Can you work these out from the model? Positions are in its coordinate system, mm. A direction names the side the tool comes from. Coordinates: 2 decimals unless noted, no trailing zeros. Order: outer loops, then holes, each group sorted by start corner. A loop starts at its lowest first (then second) coordinate and runs counter-clockwise, first axis right, second up. Notation, with made-up numbers: (72, 5.25) -> (81, 5.25) arc R30 ccw to (81, 31.25) -> close; hole circle Ø7 at (41.5, 2). An arc over 180 degrees is marked (long way). Use a Markdown table: item, result. Add a question column.
1. If I drill on line 1 along X through (y, z) = (46.5, -4); line 2 along Z through (x, y) = (-49, 14.5); line 3 along Z through (x, y) = (-22, 29), over which ranges is the centre line in solid material (lowest first)? Write a range as from..to.
2. We'd pull the mould along Y, two halves only. Please class faces 6 (the flat face through (-11, 0, -11)), 7 (the flat face through (49.429, 25, -9)), 8 (the flat face through (-22.3, 28.2, -58.583)): pulls with the +Y half, pulls with the -Y half, needs draft (parallel to the pull), parting line crosses it, or undercut.
3. For faces 1 (the flat face through (-70.571, 25, -9)), 2 (the cylindrical face through (-13.173, 12.785, -59.322)), 3 (the flat face through (-11, 25, 39.917)), 4 (the flat face through (-66.571, 27, -9)), 5 (the flat face through (-11, 40, -57)), which set-ups out of +Z, -Z, +X, -X, +Y, -Y let a thin tool reach every point of the face, with its end or its side?
4. Suppose I cut it at A-A, the plane x = 11.5. List the corners of the cut face in (y, z) for me.
5. For pin 1 Ø1.5 at (x, y) = (30.5, 26.5) entering from -Z; pin 2 Ø2 at (x, z) = (-55.5, -14) entering from +Y; pin 3 Ø1.5 at (x, z) = (-49, 17.5) entering from +Y, each with a flat end and sliding along its axis, tell me the tip position at first contact or that it passes through.
6. Suppose I cut it at B-B, the plane y = 23. List the corners of the cut face in (x, z) for me, then the cut area to 3 significant figures.
7. Suppose I cut it at D-D, the plane x = -14. List the corners of the cut face in (y, z) for me, then the cut area to 3 significant figures.
8. Suppose I cut it at C-C, the plane z = -38. List the corners of the cut face in (x, y) for me.
```python
from build123d import *

# Parameters (mm, degrees)
SKETCH1_W           = 120
SKETCH1_H           = 100
BOSS_EXTRUDE1_DEPTH = 50
SKETCH2_W           = 112
SKETCH2_H           = 92
CUT_EXTRUDE1_DEPTH  = 46
SKETCH3_W           = 28
SKETCH3_H           = 70
BOSS_EXTRUDE3_DEPTH = 8
SKETCH6_W           = 24.21
SKETCH6_H           = 8
CUT_EXTRUDE4_DEPTH  = 66
CUT_EXTRUDE6_DEPTH  = 66
SKETCH8_W           = 26
SKETCH8_H           = 31
CUT_EXTRUDE7_DEPTH  = 2.5
SKETCH9_R           = 12
CUT_EXTRUDE8_DEPTH  = 2.5
SKETCH10_R          = 7
CUT_EXTRUDE9_DEPTH  = 12.5


with BuildPart() as part:
    # Sketch1 → Boss-Extrude1 (new body)
    with BuildSketch(Plane(origin=(0, 0, 0), x_dir=(1, 0, 0), z_dir=(0, 1, 0))):
        with Locations((-10.571222942, 10.082692781)):
            Rectangle(SKETCH1_W, SKETCH1_H)
    extrude(amount=BOSS_EXTRUDE1_DEPTH)

    # Sketch2 → Cut-Extrude1 (cut)
    with BuildSketch(Plane(origin=(0, 50, 0), x_dir=(1, 0, 0), z_dir=(0, 1, 0))):
        with Locations((-10.571222942, 10.082692781)):
            Rectangle(SKETCH2_W, SKETCH2_H)
    extrude(amount=-CUT_EXTRUDE1_DEPTH, mode=Mode.SUBTRACT)

    # Sketch3 → Boss-Extrude3 (add)
    with BuildSketch(Plane(origin=(0, 4, 0), x_dir=(1, 0, 0), z_dir=(0, 1, 0))):
        with Locations((-42.571222942, 25.082692781)):
            Rectangle(SKETCH3_W, SKETCH3_H)
    extrude(amount=BOSS_EXTRUDE3_DEPTH)

    # Sketch6 → Cut-Extrude4 (cut)
    with BuildSketch(Plane.XY.offset(9.917307219)):
        with Locations((-42.569304131, 8)):
            Rectangle(SKETCH6_W, SKETCH6_H)
    extrude(amount=-CUT_EXTRUDE4_DEPTH, mode=Mode.SUBTRACT)

    # Sketch7 → Cut-Extrude6 (cut)
    with BuildSketch(Plane.XY.offset(-56.082692781)):
        Polygon((-54.674304131, 12), (-50.474304131, 12), (-50.474304131, 6.53), (-47.074304131, 6.53), (-47.074304131, 12), (-38.074304131, 12), (-38.074304131, 6.53), (-34.664304131, 6.53), (-34.664304131, 12), (-30.464304131, 12), (-30.464304131, 6.53), (-30.464304131, 4), (-54.674304131, 4), (-54.674304131, 6.53), align=None)
    extrude(amount=-CUT_EXTRUDE6_DEPTH, mode=Mode.SUBTRACT)

    # Sketch8 → Cut-Extrude7 (cut)
    with BuildSketch(Plane.XY.offset(-56.082692781)):
        with Locations((-10.571222942, 24.5)):
            Rectangle(SKETCH8_W, SKETCH8_H)
    extrude(amount=-CUT_EXTRUDE7_DEPTH, mode=Mode.SUBTRACT)

    # Sketch9 → Cut-Extrude8 (cut)
    with BuildSketch(Plane.XY.offset(-58.582692781)):
        with Locations((-10.571222942, 24.5)):
            Circle(SKETCH9_R)
    extrude(amount=-CUT_EXTRUDE8_DEPTH, mode=Mode.SUBTRACT)

    # Sketch10 → Cut-Extrude9 (cut)
    with BuildSketch(Plane(origin=(0, 0, -60.082692781), x_dir=(-1, 0, 0), z_dir=(0, 0, -1))):
        with Locations((-27.728777058, 25)):
            Circle(SKETCH10_R)
    extrude(amount=-CUT_EXTRUDE9_DEPTH, mode=Mode.SUBTRACT)


solid = part.part
```
Worked out:
| question | item | result |
|---|---|---|
| 1 | line 1 | x = -70.57..-66.57, 45.43..49.43 |
| 1 | line 2 | z = -60.08..-56.08, 35.92..39.92 |
| 1 | line 3 | z = -60.08..-58.58, 35.92..39.92 |
| 2 | face 6 | pulls with the -Y half |
| 2 | face 7 | needs draft |
| 2 | face 8 | undercut |
| 3 | face 1 | +Z, -Z, -X, +Y, -Y |
| 3 | face 2 | -Z |
| 3 | face 3 | +Z, +X, -X, +Y, -Y |
| 3 | face 4 | +Y |
| 3 | face 5 | none |
| 4 | outline | (0, -60.08) -> (50, -60.08) -> (50, -56.08) -> (4, -56.08) -> (4, 35.92) -> (50, 35.92) -> (50, 39.92) -> (0, 39.92) -> close |
| 5 | pin 1 | stops at z = 35.92 |
| 5 | pin 2 | stops at y = 12 |
| 5 | pin 3 | stops at y = 4 |
| 6 | outline | (-70.57, -60.08) -> (-22.48, -60.08) -> (-22.48, -58.58) -> (-23.57, -58.58) -> (-23.57, -56.08) -> (-66.57, -56.08) -> (-66.57, 35.92) -> (45.43, 35.92) -> (45.43, -56.08) -> (34.44, -56.08) -> (34.44, -60.08) -> (49.43, -60.08) -> (49.43, 39.92) -> (-70.57, 39.92) -> close; (1.33, -60.08) -> (21.02, -60.08) -> (21.02, -56.08) -> (2.43, -56.08) -> (2.43, -58.58) -> (1.33, -58.58) -> close |
| 6 | area | 1,540 mm² |
| 7 | outline | (0, -60.08) -> (13, -60.08) -> (13, -58.58) -> (9, -58.58) -> (9, -56.08) -> (4, -56.08) -> (4, 35.92) -> (50, 35.92) -> (50, 39.92) -> (0, 39.92) -> close; (36, -60.08) -> (50, -60.08) -> (50, -56.08) -> (40, -56.08) -> (40, -58.58) -> (36, -58.58) -> close |
| 7 | area | 656 mm² |
| 8 | outline | (-70.57, 0) -> (49.43, 0) -> (49.43, 50) -> (45.43, 50) -> (45.43, 4) -> (-28.57, 4) -> (-28.57, 12) -> (-30.46, 12) -> (-30.46, 4) -> (-54.67, 4) -> (-54.67, 12) -> (-56.57, 12) -> (-56.57, 4) -> (-66.57, 4) -> (-66.57, 50) -> (-70.57, 50) -> close |
